Input: dimensioned drawing with shaded views. Units: mm. Origin: part minimum x, y, z. A direction names the side the tool comes from. Coordinates: 2 decimals unless noted, no trailing zeros. Write each loop counter-clockwise with the first axis right and the second up, starting at its lowest first coordinate (ties: lowest second). Pieces come first, ordered by that corner, then holes. Notation, with made-up numbers: (-8, 74) -> (35, 74) arc R21 cw to (35, 112) -> close; hole circle Ø1 at (88, -32). An arc over 180 degrees is marked (long way). One line per item, written item: value. Start each with the question number.
1. Section query C-C, the plane z = 3.1. Output: boundary loops of the cut face in (x, y).
2. Line query: line 1 (Y direction, x = 11.1, z = 1.15); line 2 (Y direction, x = 11.25, z = 0.2); line 3 (Z direction, x = 15, y = 19.75). Output: solid intervals per line, ascending.
3. Mould query, pull axis Y, two halves, no side actions, for the marked faces 3, 4 and 5. Classes: released by +Y, released by -Y, zero draft, split by the parting line, or undercut.
4. Access query for the marked faces 1 and 2. Directions: +Z, -Z, +X, -X, +Y, -Y. A direction counts if a zero-diameter tool reaches every point of the face in a straight line with its end or side. Return the directions, or none.
5. Section query A-A, the plane x = 11.1. Output: boundary loops of the cut face in (y, z).
6. First-contact query: P1, Ø2, axis at x = 4, y = 16.5, coming from the +Z side; P2, Ø9, axis at x = 11.1, y = 11.1, coming from the +Z side. Flat tips, straight axial feed; report the tip coordinate or a pass-through.
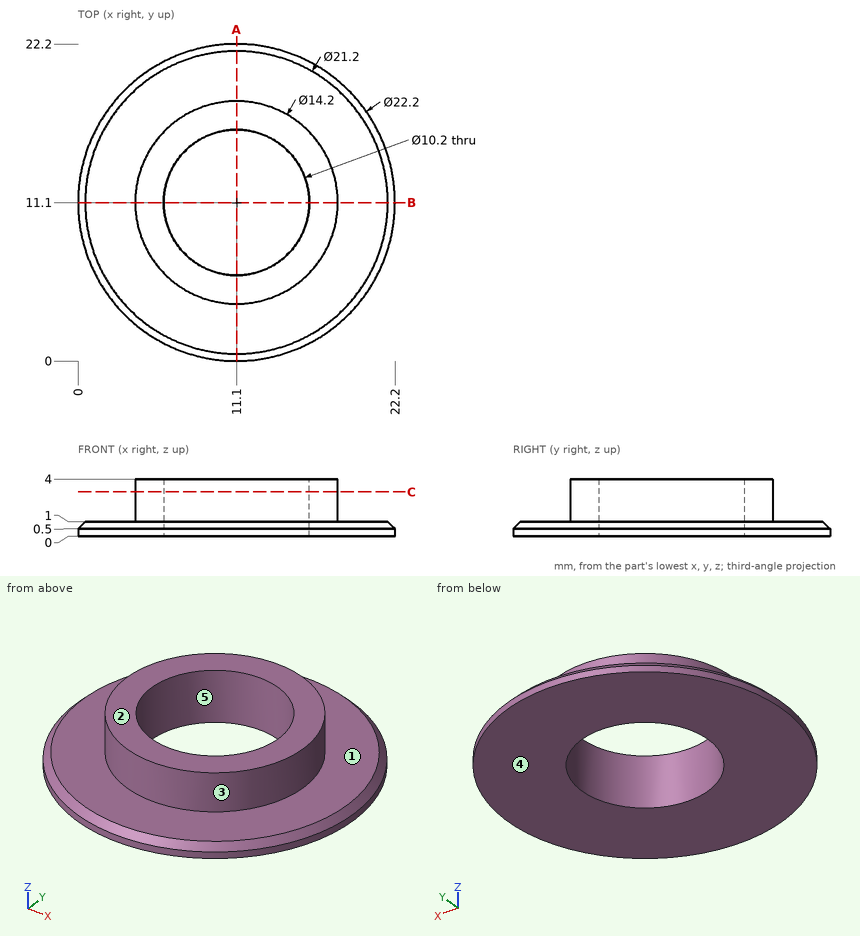
Computed values:
1. outline: circle Ø14.2 at (11.1, 11.1); hole circle Ø10.2 at (11.1, 11.1)
2. line 1: y = 4 to 6, 16.2 to 18.2
2. line 2: y = 0 to 6, 16.2 to 22.2
2. line 3: z = 0 to 1
3. face 3: split by the parting line
3. face 4: zero draft
3. face 5: undercut
4. face 1: +Z
4. face 2: +Z, +X, -X, +Y, -Y
5. outline: (0, 0) -> (6, 0) -> (6, 4) -> (4, 4) -> (4, 1) -> (0.5, 1) -> (0, 0.5) -> close; (16.2, 0) -> (22.2, 0) -> (22.2, 0.5) -> (21.7, 1) -> (18.2, 1) -> (18.2, 4) -> (16.2, 4) -> close
6. P1: stops at z = 1
6. P2: passes through
